Check sheet for the modelled part. Datum: model origin and axes. Units: mm. Face numbers are marked on the shaded views. A direction names the side the tool comes from. Round coordinates to 2 decimals unless told otherwise and drop trailing zeros. Write each loop counter-clockwise with the first axis right and the second up, starting at its lowest first coordinate (ties: lowest second). Pieces come first, ordered by that corner, then holes.
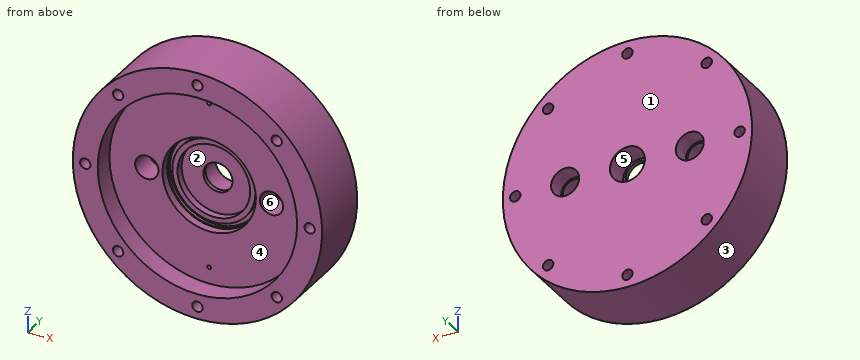
from build123d import *

# Parameters (mm, degrees)
SKETCH1_R                                      = 76.2
BILLET_DEPTH                                   = 50.8
SKETCH3_R                                      = 28.575
LOX_PLATE_DEPTH                                = 17.78
SKETCH5_R                                      = 22.225
LOX_DOME_DEPTH                                 = 4.46278
SKETCH7_R                                      = 76.2
TOP_MILL_DEPTH                                 = 12.7
F_1_4_BOLT_HOLE_REACH                          = 116.3
SKETCH11_R                                     = 3.175
BOLT_PATTERN_COUNT                             = 8
SKETCH12_R                                     = 60.96
KEROSENE_PLATE_DEPTH                           = 12.7
SKETCH26_R                                     = 27.94
SKETCH26_R_2                                   = 25.4
LOX_PLATE_O_RING_DEPTH                         = 2.032
KEROSENE_INLET_3_8_NPT_TAPPED_HOLE1_AT_2_COUNT = 2
KEROSENE_INLET_3_8_NPT_TAPPED_HOLE1_AT_2_PITCH = 76.2
SKETCH27_R                                     = 1.190625
CUT_EXTRUDE1_DEPTH                             = 3.175


with BuildPart() as part:
    # Sketch1 → Billet (new body)
    with BuildSketch(Plane(origin=(0, 0, 0), x_dir=(1, 0, 0), z_dir=(0, 1, 0))):
        with Locations(Location((0, 0, 0), (0, 0, 270))):
            Circle(SKETCH1_R)
    extrude(amount=-BILLET_DEPTH)

    # Sketch3 → Lox Plate (cut)
    with BuildSketch(Plane(origin=(0, -50.8, 0), x_dir=(1, 0, 0), z_dir=(0, 1, 0))):
        with Locations(Location((0, 0, 0), (0, 0, 270))):
            Circle(SKETCH3_R)
    extrude(amount=LOX_PLATE_DEPTH, mode=Mode.SUBTRACT)

    # Sketch5 → Lox Dome (cut)
    with BuildSketch(Plane(origin=(0, -33.02, 0), x_dir=(1, 0, 0), z_dir=(0, 1, 0))):
        with Locations(Location((0, 0, 0), (0, 0, 270))):
            Circle(SKETCH5_R)
    extrude(amount=LOX_DOME_DEPTH, mode=Mode.SUBTRACT)

    # Sketch7 → Top Mill (cut)
    with BuildSketch(Plane(origin=(0, 0, 0), x_dir=(1, 0, 0), z_dir=(0, 1, 0))):
        with Locations(Location((0, 0, 0), (0, 0, 270))):
            Circle(SKETCH7_R)
    extrude(amount=-TOP_MILL_DEPTH, mode=Mode.SUBTRACT)

    # Sketch11 → 1_4_ Bolt Hole (cut, up to next)
    with BuildSketch(Plane(origin=(0, -50.8, 0), x_dir=(1, 0, 0), z_dir=(0, 1, 0)), mode=Mode.PRIVATE) as f_1_4_bolt_hole_sk1:
        with Locations(Location((0, 68.58, 0), (0, 0, 270))):
            Circle(SKETCH11_R)
    f_1_4_bolt_hole_tool1 = extrude(f_1_4_bolt_hole_sk1.sketch, amount=F_1_4_BOLT_HOLE_REACH, mode=Mode.PRIVATE) & part.part
    f_1_4_bolt_hole = f_1_4_bolt_hole_tool1.solids().sort_by_distance((0, -50.8, -68.58))[0]
    add(f_1_4_bolt_hole, mode=Mode.SUBTRACT)

    # Bolt Pattern: 1_4_ Bolt Hole ×8 about axis
    bolt_pattern_axis = Axis((0, 0, 0), (0, 1, 0))
    for i in range(1, BOLT_PATTERN_COUNT):
        add(f_1_4_bolt_hole.rotate(bolt_pattern_axis, i * 360 / BOLT_PATTERN_COUNT), mode=Mode.SUBTRACT)

    # Sketch12 → Kerosene Plate (cut)
    with BuildSketch(Plane(origin=(0, -50.8, 0), x_dir=(1, 0, 0), z_dir=(0, 1, 0))):
        with Locations(Location((0, 0, 0), (0, 0, 270))):
            Circle(SKETCH12_R)
    extrude(amount=KEROSENE_PLATE_DEPTH, mode=Mode.SUBTRACT)

    # Sketch21 → Lox Inlet-1_2 NPT Tapped Hole3 (revolve, cut)
    with BuildSketch(Plane(origin=(0, -12.7, 0), x_dir=(0, 0, 1), z_dir=(1, 0, 0))):
        Polygon((0, 0), (0, 38.1), (8.9281, 38.1), (8.9281, 13.462), (10.261665792, 13.462), (10.6647361, 0), align=None)
    revolve(axis=Axis((0, -6.35, 0), (0, -1, 0)), mode=Mode.SUBTRACT)

    # Sketch26 → Lox Plate O Ring (cut)
    with BuildSketch(Plane.XZ.offset(33.02)):
        with Locations(Location((0, 0, 0), (0, 0, 270))):
            Circle(SKETCH26_R)
        with Locations(Location((0, 0, 0), (0, 0, 270))):
            Circle(SKETCH26_R_2, mode=Mode.SUBTRACT)
    extrude(amount=-LOX_PLATE_O_RING_DEPTH, mode=Mode.SUBTRACT)

    # Sketch25 → Kerosene Inlet-3_8 NPT Tapped Hole1 (revolve, cut)
    with BuildSketch(Plane(origin=(-38.1, -12.7, 0), x_dir=(0, 0, 1), z_dir=(1, 0, 0))):
        Polygon((0, 0), (0, 38.1), (7.1374, 38.1), (7.1374, 10.414), (8.263205494, 10.414), (8.5750146, 0), align=None)
    kerosene_inlet_3_8_npt_tapped_hole1 = revolve(axis=Axis((-38.1, -6.35, 0), (0, -1, 0)), mode=Mode.SUBTRACT)

    # Kerosene Inlet-3_8 NPT Tapped Hole1 at 2: Kerosene Inlet-3_8 NPT Tapped Hole1 ×2
    with Locations(*[(i * KEROSENE_INLET_3_8_NPT_TAPPED_HOLE1_AT_2_PITCH, 0, 0) for i in range(1, KEROSENE_INLET_3_8_NPT_TAPPED_HOLE1_AT_2_COUNT)]):
        add(kerosene_inlet_3_8_npt_tapped_hole1, mode=Mode.SUBTRACT)

    # Sketch27 → Cut-Extrude1 (cut)
    with BuildSketch(Plane.XZ.offset(38.1)):
        with Locations(Location((0, 50.8, 0), (0, 0, 270))):
            Circle(SKETCH27_R)
        with Locations(Location((0, -50.8, 0), (0, 0, 90))):
            Circle(SKETCH27_R)
    extrude(amount=-CUT_EXTRUDE1_DEPTH, mode=Mode.SUBTRACT)


solid = part.part
1. Set-up check for the marked faces 4, 5 and 6: record each of +Z, -Z, +X, -X, +Y, -Y from which the full face is reachable in a straight line by a thin tool's end or side.
2. Sectioned sample at A-A, the plane z = -68.58. Enter the section's corners in (x, y) (3 decimals), plus the area to 3 significant figures.
3. Sectioned sample at C-C, the plane y = -20. Give the number of separate pieces and of enclosed holes in the cut face, plus the area to 3 significant figures.
4. Go/stop test with flat-tipped pins: pin 1 (8.5 mm diameter, centred on x = 38.5, z = 0, fed in from +Y); pin 2 (12 mm diameter, centred on x = -23, y = -26.5, fed in from -Z); pin 3 (8 mm diameter, centred on y = -21, z = 28.5, fed in from +X); pin 4 (4 mm diameter, centred on x = -37.5, y = -45, fed in from -Z). Record where each tip stops, or that it passes through.
5. Release check for a two-part mould opening along Z. For the marked faces 1, 2 and 3 record: released by +Z, released by -Z, zero draft, split by the parting line, or undercut.
6. Scan lines: line 1 along X through (y, z) = (-25, 46.5); line 2 along X through (y, z) = (-39, 13); line 3 along Z through (x, y) = (-38.1, -33.25). Record each from-to range of solid material in increasing order.
7. Sectioned sample at B-B, the plane x = 38.1. Enter the section's corners in (y, z), plus the area to 3 significant figures.
Computed values:
1. face 4: -Y
1. face 5: +Y
1. face 6: +Y, -Y
2. outline: (-33.215, -50.8) - (-3.175, -50.8) - (-3.175, -12.7) - (-33.215, -12.7) - close; (3.175, -50.8) - (33.215, -50.8) - (33.215, -12.7) - (3.175, -12.7) - close
2. area: 2,290 mm2
3. separate pieces: 1
3. enclosed holes: 11
3. area: 17,200 mm2
4. pin 1: passes through
4. pin 2: stops at z = -74.28
4. pin 3: stops at x = 72.15
4. pin 4: stops at z = -67.43
5. face 1: zero draft
5. face 2: undercut
5. face 3: split by the parting line
6. line 1: x = -60.37 to -50.96, -46.02 to 46.02, 50.96 to 60.37
6. line 2: x = -75.08 to -59.56, 59.56 to 75.08
6. line 3: z = -65.99 to -7.14, 7.14 to 65.99
7. outline: (-50.8, -65.99) - (-12.7, -65.99) - (-12.7, -8.58) - (-23.11, -8.26) - (-23.11, -7.14) - (-38.1, -7.14) - (-38.1, -47.59) - (-50.8, -47.59) - close; (-50.8, 47.59) - (-38.1, 47.59) - (-38.1, 7.14) - (-23.11, 7.14) - (-23.11, 8.26) - (-12.7, 8.58) - (-12.7, 65.99) - (-50.8, 65.99) - close
7. area: 3,430 mm2
